Source: CAD feature listing. Evaluate the final solid. Frame: model axes, mm. A direction names the side the tool comes from. Round coordinates to 2 decimals unless told otherwise and drop trailing zeros. Loops run counter-clockwise (first coordinate to the right, second up) from the corner with the lowest first, then second, coordinate; pieces in that order, holes last. Notation, with made-up numbers: (55, 34) - (66, 34) arc R19 cw to (66, 55) - close; hole circle Ø8 at (-7, -8.75). An arc over 180 degrees is marked (long way). Use CSV: the item, a comma, the result in double quotes. Start each with the question number.
from build123d import *

# Parameters (mm, degrees)
CUT_EXTRUDE1_DEPTH  = 10
SKETCH4_R           = 1.75
BOSS_EXTRUDE1_DEPTH = 7
CUT_EXTRUDE2_DEPTH  = 3


with BuildPart() as part:
    # Sketch1 → Revolve1 (revolve)
    with BuildSketch(Plane.XY, mode=Mode.PRIVATE) as revolve1_sk:
        Polygon((0, 12), (15.4, 12), (15.4, 0), (16.9, 0), (16.9, 24.8), (16.5, 24.8), (16.5, 26.5), (15.4, 26.5), (15.4, 19.5), (0, 19.5), align=None)
    revolve(revolve1_sk.sketch.rotate(Axis((0, 0, 0), (0, 1, 0)), 90), axis=Axis((0, 0, 0), (0, 1, 0)))

    # Sketch3 → Cut-Extrude1 (cut)
    with BuildSketch(Plane.XY.offset(16.9)):
        with BuildLine():
            Line((-4, 26.5), (-4, 23.5))
            ThreePointArc((-4, 23.5), (0, 19.5), (4, 23.5))
            Line((4, 23.5), (4, 26.5))
            Line((4, 26.5), (-4, 26.5))
        make_face()
    extrude(amount=-CUT_EXTRUDE1_DEPTH, mode=Mode.SUBTRACT)

    # Sketch4 → Boss-Extrude1 (add)
    with BuildSketch(Plane(origin=(0, 24.8, 0), x_dir=(1, 0, 0), z_dir=(0, 1, 0))):
        with BuildLine():
            Line((21, -4), (16.419805115, -4))
            ThreePointArc((16.419805115, -4), (16.9, 0), (16.419805115, 4))
            Line((16.419805115, 4), (21, 4))
            ThreePointArc((21, 4), (25, 0), (21, -4))
        make_face()
        with Locations(Location((21, 0, 0), (0, 0, 270))):
            Circle(SKETCH4_R, mode=Mode.SUBTRACT)
    boss_extrude1 = extrude(amount=-BOSS_EXTRUDE1_DEPTH)

    # Sketch5 → Cut-Extrude2 (cut)
    with BuildSketch(Plane.XZ.offset(-17.8)):
        Polygon((18.35, -1.529978213), (21, -3.059956427), (23.65, -1.529978213), (23.65, 1.529978213), (21, 3.059956427), (18.35, 1.529978213), align=None)
    cut_extrude2 = extrude(amount=-CUT_EXTRUDE2_DEPTH, mode=Mode.SUBTRACT)

    # Mirror1: Boss-Extrude1, Cut-Extrude2 across plane
    add(boss_extrude1.mirror(Plane(origin=(0, 0, 0), x_dir=(0, 0, 1), z_dir=(1, 0, 0))))
    add(cut_extrude2.mirror(Plane(origin=(0, 0, 0), x_dir=(0, 0, 1), z_dir=(1, 0, 0))), mode=Mode.SUBTRACT)


solid = part.part
1. Line query: line 1 along X through (y, z) = (24.25, 0); line 2 along Z through (x, y) = (-21, 23.4); line 3 along Y through (x, z) = (10.5, -13). Output: solid intervals per line, ascending.
2. Contact query for flat-ended pins moving along their axis: P1, Ø1, axis at y = 14.5, z = -13, coming from the -X side; P2, Ø0.5, axis at y = 25.5, z = 15.5, coming from the +X side; P3, Ø4.5, axis at x = -21, z = 0, coming from the -Y side. Output: stop coordinate, or through.
3. Mould query, pull axis Z, two halves, no side actions, for faces 1 (the flat face through (-4, 25, 15.7)), 2 (the flat face through (-19, 21, -4)), 3 (the cylindrical face through (-22.735, 22.828, -0.228)). Classes: +Z half, -Z half, draft (parallel to the pull), parting line (faces both ways), or undercut.
4. Section query C-C on y = 11. Return the cut outline in (x, z), and give its area (3 significant figures).
5. Section query A-A on x = 20. Return the cut outline in (y, z), and give its area (3 significant figures).
6. Section query D-D on x = -5.5. Return the cut outline in (y, z).
7. Reachability of faces 4 (the flat face through (18.35, 19, 0)), 5 (the flat face through (19, 21, 4)), 6 (the flat face through (0, 19.5, 0)), 7 (the flat face through (19, 21, -4)), 8 (the cylindrical face through (-25, 21, 0)) from +Z, -Z, +X, -X, +Y, -Y: full face, straight path, thin tool, end or side. Return the list, or none.
8. Section query B-B on z = 0. Give the number of separate pieces and of enclosed holes in the cut face, and give its area (3 significant figures).
Values:
1,line 1,"x = -25 to -22.75, -19.25 to -15.4, 15.4 to 19.25, 22.75 to 25"
1,line 2,"z = -4 to -1.75, 1.75 to 4"
1,line 3,"y = 0 to 24.8"
2,P1,"stops at x = -11.37"
2,P2,"stops at x = 6.3"
2,P3,"stops at y = 20.8"
3,face 1,"draft"
3,face 2,"-Z half"
3,face 3,"undercut"
4,outline,"circle Ø33.8 at (0, 0); hole circle Ø30.8 at (0, 0)"
4,area,"152 mm^2"
5,outline,"(17.8, -4) - (24.8, -4) - (24.8, -1.44) - (20.8, -1.44) - (20.8, -2.48) - (17.8, -2.48) - close; (17.8, 2.48) - (20.8, 2.48) - (20.8, 1.44) - (24.8, 1.44) - (24.8, 4) - (17.8, 4) - close"
5,area,"29.6 mm^2"
6,outline,"(0, -15.98) - (24.8, -15.98) - (24.8, -15.56) - (26.5, -15.56) - (26.5, -14.38) - (19.5, -14.38) - (19.5, 14.38) - (26.5, 14.38) - (26.5, 15.56) - (24.8, 15.56) - (24.8, 15.98) - (0, 15.98) - (0, 14.38) - (12, 14.38) - (12, -14.38) - (0, -14.38) - close"
7,face 4,"-Y"
7,face 5,"+Z, +X, +Y, -Y"
7,face 6,"+Y"
7,face 7,"-Z, +X, +Y, -Y"
7,face 8,"-X, +Y, -Y"
8,separate pieces,"3"
8,enclosed holes,"0"
8,area,"363 mm^2"
